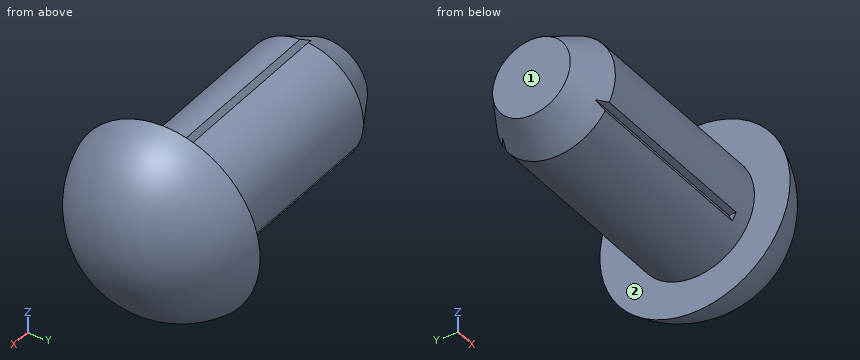
from build123d import *

# Parameters (mm, degrees)
CUT_EXTRUDE1_DEPTH = 37
CIRPATTERN1_COUNT  = 3


with BuildPart() as part:
    # Sketch1 → Base-Revolve (revolve)
    with BuildSketch(Plane.XY, mode=Mode.PRIVATE) as base_revolve_sk:
        with BuildLine():
            Line((-40, 0), (-40, 6.535898385))
            Line((-40, 6.535898385), (-34, 10))
            Line((-34, 10), (0, 10))
            Line((0, 10), (0, 16))
            ThreePointArc((0, 16), (8.983547964, 10.142395515), (12.468871126, 0))
            Line((12.468871126, 0), (-40, 0))
        make_face()
    revolve(base_revolve_sk.sketch.rotate(Axis((-40, 0, 0), (1, 0, 0)), 90), axis=Axis((-40, 0, 0), (1, 0, 0)))

    # Sketch2 → Cut-Extrude1 (cut)
    with BuildSketch(Plane.ZY.offset(40)):
        Polygon((9, 0), (10, 0.700207538), (10, -0.700207538), align=None)
    cut_extrude1 = extrude(amount=-CUT_EXTRUDE1_DEPTH, mode=Mode.SUBTRACT)

    # CirPattern1: Cut-Extrude1 ×3 about axis
    cirpattern1_axis = Axis((0, 0, 0), (1, 0, 0))
    for i in range(1, CIRPATTERN1_COUNT):
        add(cut_extrude1.rotate(cirpattern1_axis, i * 360 / CIRPATTERN1_COUNT), mode=Mode.SUBTRACT)


solid = part.part
Source: CAD feature listing. Evaluate the final solid. Frame: model axes, mm. Face numbers are marked on the shaded views. A direction names the side the tool comes from. Give positions to 0.01 mm unless a question says otherwise; leave off trailing zeros. Write each loop counter-clockwise with the first axis right and the second up, starting at its lowest first coordinate (ties: lowest second). Pieces come first, ordered by that corner, then holes. Notation, with made-up numbers: (35, 28) -> (53, 28) arc R20 cw to (53, 53) -> close; hole circle Ø6 at (-10.5, 20). An arc over 180 degrees is marked (long way). Return JSON: item names as keys, results as strings. Group by question number.
1. Section C-C, the plane x = -2. Output: boundary loops of the cut face in (y, z).
2. Material intervals for line 1 (Y direction, x = -21, z = 0); line 2 (Y direction, x = -4, z = 4); line 3 (X direction, y = -8, z = -1), sorted ascending. Write a range as from..to.
3. Pin query (flat end, axial travel): pin 1 Ø0.6 at (y, z) = (-8, -5) entering from -X; pin 2 Ø6 at (x, z) = (-14, 0.5) entering from +Y; pin 3 Ø12 at (y, z) = (3, 11) entering from +X; pin 4 Ø2 at (x, y) = (-31.5, -12.5) entering from +Z. Return the tip coordinate at first contact, or that it passes through.
4. Section B-B, the plane x = -16.5. Output: boundary loops of the cut face in (y, z), then the cut area to 3 significant figures.
5. Section A-A, the plane z = 0. Output: boundary loops of the cut face in (x, y), then the cut area to 3 significant figures.
6. Access query for the marked faces 1 and 2. Directions: +Z, -Z, +X, -X, +Y, -Y. A direction counts if a zero-diameter tool reaches every point of the face in a straight line with its end or side. Return the directions, or none.
Determined:
{
 "1": {"outline": "circle Ø20 at (0, 0)"},
 "2": {"line 1": "y = -10..10", "line 2": "y = -9.17..9.17", "line 3": "x = -37.36..10.37"},
 "3": {"pin 1": "stops at x = -35.5", "pin 2": "stops at y = 10", "pin 3": "stops at x = 11.56", "pin 4": "passes through"},
 "4": {"outline": "(-8.98, -4.4) -> (-7.79, -4.5) -> (-8.3, -5.58) arc R10 ccw to (8.3, -5.58) -> (7.79, -4.5) -> (8.98, -4.4) arc R10 ccw to (0.68, 9.98) -> (0, 9) -> (-0.68, 9.98) arc R10 ccw to start", "area": "312 mm2"},
 "5": {"outline": "(-40, -6.54) -> (-34, -10) -> (0, -10) -> (0, -16) arc R16.5 ccw to (0, 16) -> (0, 10) -> (-34, 10) -> (-40, 6.54) -> close", "area": "1,080 mm2"},
 "6": {"face 1": "+Z, -Z, -X, +Y, -Y", "face 2": "-X"}
}
